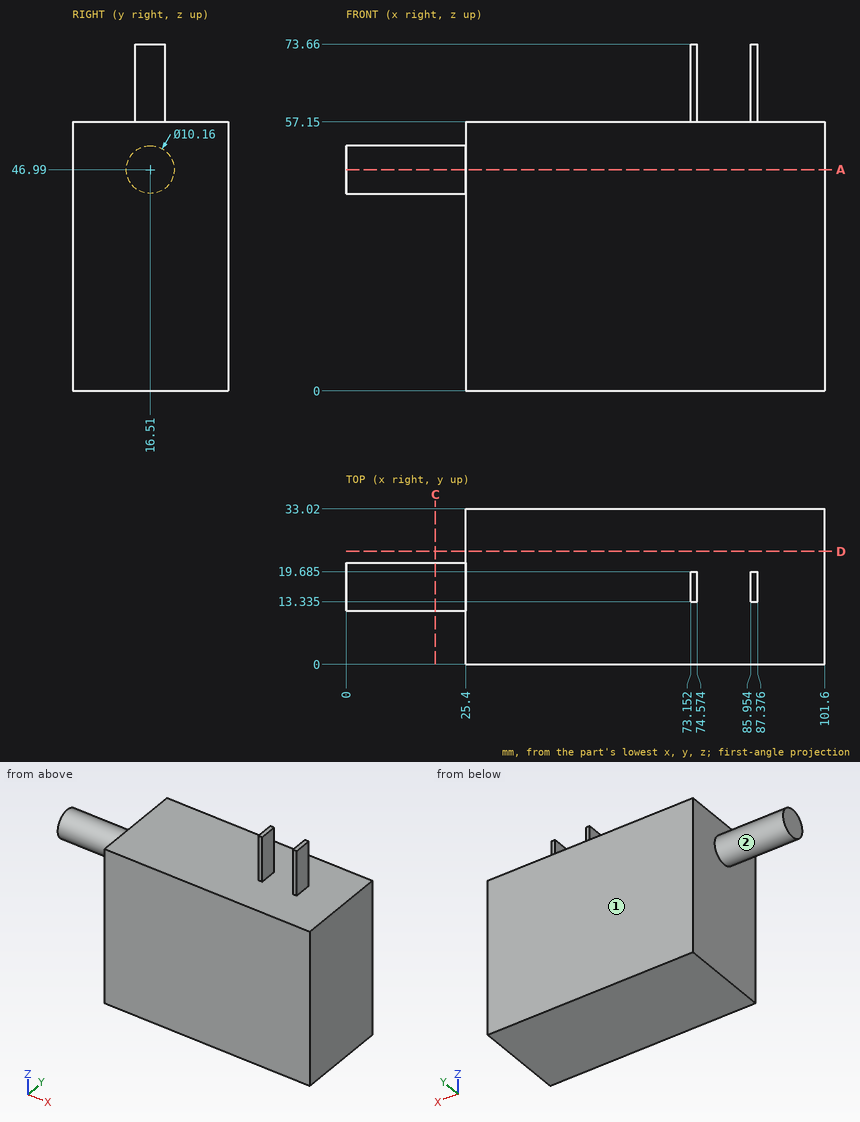
Can you work these out from the drawing? Everything is in mm from the part's minimum corner. A direction names the side the tool comes from. Round coordinates to 2 decimals unless told otherwise and drop trailing zeros. Loops run counter-clockwise (first coordinate to the right, second up) from the corner with the lowest first, then second, coordinate; pieces in that order, holes last. Notation, with made-up numbers: (-7, -35.5) - (1, -35.5) arc R20 cw to (1, -10.5) - close; hole circle Ø1 at (59, -8.75). An arc over 180 degrees is marked (long way). Answer in a Markdown table with one row per item. Add a question column.
(1) If we section it at D-D (y = 24): Please give me the cut outline in (x, z).
(2) I'm going to push flat-ended pins straight in: pin 1 (0.7 mm diameter, centred on x = 86.5, z = 63, fed in from -Y) (3 decimals); pin 2 (2 mm diameter, centred on x = 77.5, y = 10, fed in from +Z); pin 3 (2 mm diameter, centred on x = 62.5, z = 49.5, fed in from -Y); pin 4 (3 mm diameter, centred on y = 17.5, z = 67, fed in from -X). Where does each tip first touch, or does it pass through?
(3) For the marked faces 1 and 2, which set-ups out of +Z, -Z, +X, -X, +Y, -Y let a thin tool reach every point of the face, with its end or its side?
(4) I need wall thicknesses on line 1 along X through (y, z) = (10, 45.5); line 2 along Y through (x, z) = (73.5, 68) (1 decimal); line 3 along Z through (x, y) = (65.5, 21). Which ranges of each line are inside material? Lowest first, please.
(5) If we section it at C-C (x = 19): Please give me the cut outline in (y, z).
(6) If we section it at A-A (z = 46.99): Please give me the cut outline in (x, y), plus the area to 3 significant figures.
Model answer:
| question | item | result |
|---|---|---|
| 1 | outline | (25.4, 0) - (101.6, 0) - (101.6, 57.15) - (25.4, 57.15) - close |
| 2 | pin 1 | stops at y = 13.335 |
| 2 | pin 2 | stops at z = 57.15 |
| 2 | pin 3 | stops at y = 0 |
| 2 | pin 4 | stops at x = 73.15 |
| 3 | face 1 | +Z, -Z, +X, -X, +Y |
| 3 | face 2 | -X |
| 4 | line 1 | x = 25.4 to 101.6 |
| 4 | line 2 | y = 13.3 to 19.7 |
| 4 | line 3 | z = 0 to 57.15 |
| 5 | outline | circle Ø10.16 at (16.51, 46.99) |
| 6 | outline | (0, 11.43) - (25.4, 11.43) - (25.4, 0) - (101.6, 0) - (101.6, 33.02) - (25.4, 33.02) - (25.4, 21.59) - (0, 21.59) - close |
| 6 | area | 2,770 mm² |
